```python
from build123d import *

# Parameters (mm, degrees)
SKETCH017_R             = 15
PAD009_DEPTH            = 10
POCKET003_DEPTH         = 2.5
POLARPATTERN003_COUNT   = 4
SKETCH014_R             = 0.75
HOLE001_DEPTH           = 25
POLARPATTERN002_COUNT   = 4
SKETCH015_R             = 4
POCKET004_DEPTH         = 7.501
POCKET005_DEPTH         = 4.5
BODY010_PLACEMENT_ANGLE = 90


with BuildPart() as part:
    # Sketch017 → Pad009 (new body)
    with BuildSketch(Plane.XY):
        Circle(SKETCH017_R)
    extrude(amount=PAD009_DEPTH)

    # Sketch016 (on Face3 of Pad009) → Pocket003 (cut)
    with BuildSketch(Plane.XY.offset(10)):
        with BuildLine():
            ThreePointArc((-5.26869, 1.578261), (0, -5.5), (5.26869, 1.578261))
            Line((2.107476, 12.131304), (5.26869, 1.578261))
            ThreePointArc((2.107476, 12.131304), (0, 13.7), (-2.107476, 12.131304))
            Line((-2.107476, 12.131304), (-5.26869, 1.578261))
        make_face()
    pocket003 = extrude(amount=-POCKET003_DEPTH, mode=Mode.SUBTRACT)

    # PolarPattern003: Pocket003 ×4 about axis
    polarpattern003_axis = Axis((0, 0, 10), (0, 0, 1))
    for i in range(1, POLARPATTERN003_COUNT):
        add(pocket003.rotate(polarpattern003_axis, i * 360 / POLARPATTERN003_COUNT), mode=Mode.SUBTRACT)

    # Sketch014 (on Face21 of PolarPattern003) → Hole001 (cut)
    with BuildSketch(Plane.XY.offset(7.5)):
        with Locations((0, 11)):
            Circle(SKETCH014_R)
    hole001 = extrude(amount=-HOLE001_DEPTH, mode=Mode.SUBTRACT)

    # PolarPattern002: Hole001 ×4 about axis
    polarpattern002_axis = Axis((0, 0, 7.5), (0, 0, 1))
    for i in range(1, POLARPATTERN002_COUNT):
        add(hole001.rotate(polarpattern002_axis, i * 360 / POLARPATTERN002_COUNT), mode=Mode.SUBTRACT)

    # Sketch015 (on Face25 of PolarPattern002) → Pocket004 (cut, through all)
    with BuildSketch(Plane.XY.offset(7.5)):
        Circle(SKETCH015_R)
    extrude(amount=-POCKET004_DEPTH, mode=Mode.SUBTRACT)

    # Sketch018 (on Face24 of Pocket004) → Pocket005 (cut)
    with BuildSketch(Plane.XY.offset(7.5)):
        Polygon((-2.396004, 4.15), (-4.792007, 0), (-2.396004, -4.15), (2.396004, -4.15), (4.792007, 0), (2.396004, 4.15), align=None)
    extrude(amount=-POCKET005_DEPTH, mode=Mode.SUBTRACT)


with BuildPart() as part_1:
    # Body010 placement: moved
    add(part.part.moved(Location((-25, 0, 0))).rotate(Axis((-25, 0, 0), (0, -1, 0)), BODY010_PLACEMENT_ANGLE))


solid = part_1.part
```
Input: part model. Units: mm. Frame: model coordinates. A direction names the side the tool comes from. Coordinates: 2 decimals unless noted, no trailing zeros. Order: outer loops, then holes, each group sorted by start corner. A loop starts at its lowest first (then second) coordinate and runs counter-clockwise, first axis right, second up. Notation, with made-up numbers: (33, 62) - (44, 62) arc R22 cw to (44, 92) - close; hole circle Ø3 at (-28.5, 80). An arc over 180 degrees is marked (long way). Return JSON: item names as keys, results as strings.
Q1. Cut plane B-B (z = 0). Return loops of the section in (x, y), then the cut area to 3 significant figures.
The answers:
{"outline": "(-35, -15) - (-25, -15) - (-25, -11.75) - (-32.5, -11.75) - (-32.5, -13.7) - (-35, -13.7) - close; (-35, 13.7) - (-32.5, 13.7) - (-32.5, 11.75) - (-25, 11.75) - (-25, 15) - (-35, 15) - close; (-32.5, -10.25) - (-25, -10.25) - (-25, -4) - (-28, -4) - (-28, -4.15) - (-32.5, -4.15) - close; (-32.5, 4.15) - (-28, 4.15) - (-28, 4) - (-25, 4) - (-25, 10.25) - (-32.5, 10.25) - close", "area": "148 mm2"}
Q2. Cut plane D-D (x = -30.75). Return loops of the section in (y, z).
The answers:
{"outline": "circle Ø30 at (0, 0); hole circle Ø1.5 at (-11, 0); hole (-4.15, -2.4) - (0, -4.79) - (4.15, -2.4) - (4.15, 2.4) - (0, 4.79) - (-4.15, 2.4) - close; hole circle Ø1.5 at (0, -11); hole circle Ø1.5 at (0, 11); hole circle Ø1.5 at (11, 0)"}
Q3. Cut plane C-C (y = 11). Return loops of the section in (x, z), then the cut area to 3 significant figures.
The answers:
{"outline": "(-35, -10.2) - (-25, -10.2) - (-25, -0.75) - (-32.5, -0.75) - (-32.5, -2.45) - (-35, -2.45) - close; (-35, 2.45) - (-32.5, 2.45) - (-32.5, 0.75) - (-25, 0.75) - (-25, 10.2) - (-35, 10.2) - close", "area": "180 mm2"}
Q4. First-contact query: pin 1 (4 mm diameter, centred on x = -27.5, y = -8, fed in from +Z); pin 2 (1 mm diameter, centred on x = -27, z = 10.5, fed in from +Y); pin 3 (2.5 mm diameter, centred on y = 11, z = 0, fed in from -X). Flat tips, straight axial feed; report the tip coordinate or a pass-through.
The answers:
{"pin 1": "stops at z = 13.75", "pin 2": "stops at y = 11.18", "pin 3": "stops at x = -32.5"}
Q5. Ray query, probe 1 along Y at (x, z) = (-26.35, 0); probe 2 along Y at (x, z) = (-30.25, 0); probe 3 along X at (y, z) = (0, -8.5). Return the intervals inside material, ascending.
The answers:
{"probe 1": "y = -15 to -11.75, -10.25 to -4, 4 to 10.25, 11.75 to 15", "probe 2": "y = -15 to -11.75, -10.25 to -4.15, 4.15 to 10.25, 11.75 to 15", "probe 3": "x = -32.5 to -25"}
Q6. Access query for faces 3 (the cylindrical face through (-33.8, -13.7, 0)), 4 (the cylindrical face through (-28.802, 0.098, 11.744)). Directions: +Z, -Z, +X, -X, +Y, -Y. A direction counts if a zero-diameter tool reaches every point of the face in a straight line with its end or side. Return the directions, or none.
The answers:
{"face 3": "-X", "face 4": "+X, -X"}
Q7. Cut plane A-A (x = -33.25). Return loops of the section in (y, z), then the cut area to 3 significant figures.
The answers:
{"outline": "circle Ø30 at (0, 0); hole (-12.13, -2.11) - (-4.42, -4.42) - (-2.11, -12.13) arc R2.2 ccw to (2.11, -12.13) - (4.42, -4.42) - (12.13, -2.11) arc R2.2 ccw to (12.13, 2.11) - (4.42, 4.42) - (2.11, 12.13) arc R2.2 ccw to (-2.11, 12.13) - (-4.42, 4.42) - (-12.13, 2.11) arc R2.2 ccw to start", "area": "408 mm2"}
Q8. Draft query along Z for faces 1 (the flat face through (-30.28, 2.05, 3.61)), 2 (the flat face through (-35, -6, 6)). Return one class per face: +Z half, -Z half, draft (parallel to the pull), parting line (faces both ways), or undercut.
The answers:
{"face 1": "undercut", "face 2": "draft"}
